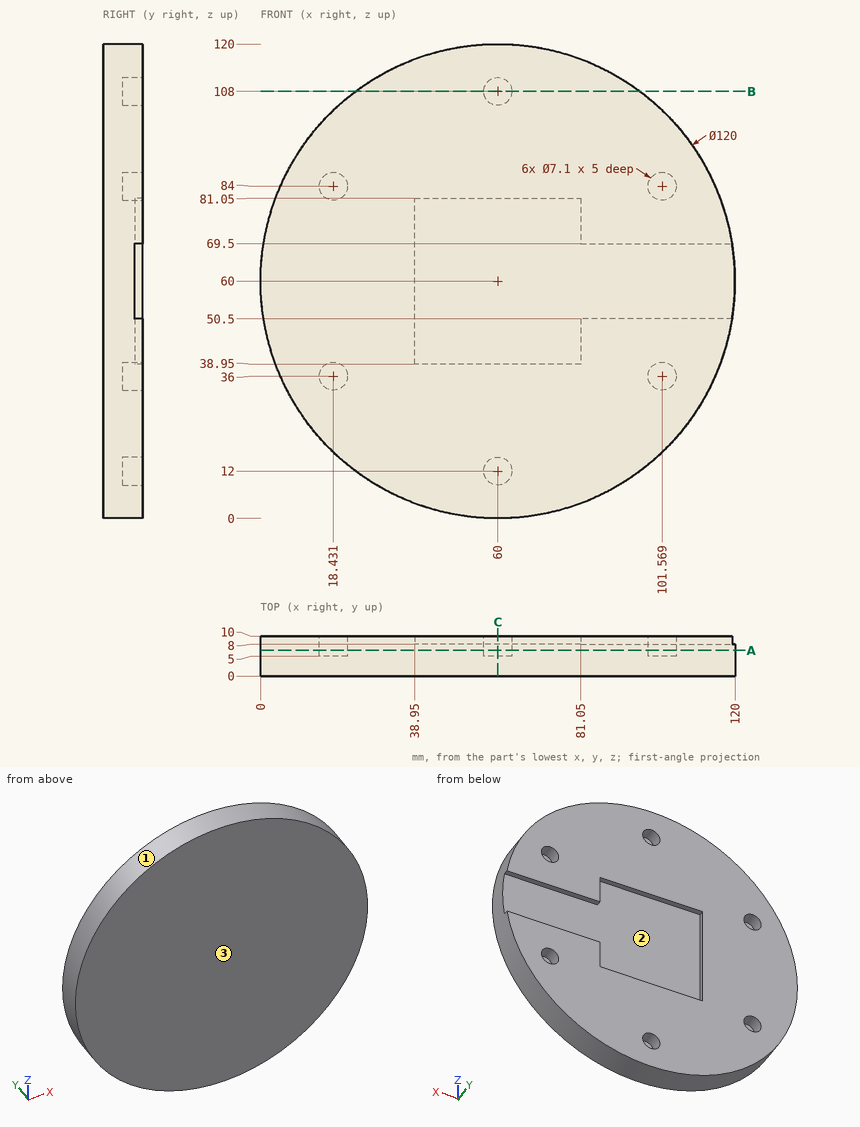
Design review of the part shown in the three views and the two pictorial views. Dimensions are in mm from the part's minimum x, y and z. Give positions to 0.01 mm unless a question says otherwise; leave off trailing zeros. Write each loop counter-clockwise with the first axis right and the second up, starting at its lowest first coordinate (ties: lowest second). Pieces come first, ordered by that corner, then holes. Notation, with made-up numbers: M -35.5,57.5 L 4.5,57.5 A27 ccw 4.5,79.5 Z; hole C 83,40 d10. An arc over 180 degrees is marked long. Answer as CSV lines item,"result".
1. Consider section A-A, the plane y = 6.5. Write out the cut boundary in (x, z), then the cut area to 3 significant figures.
Findings:
outline,"C 60,60 d120; hole C 18.43,36 d7.1; hole C 18.43,84 d7.1; hole C 60,12 d7.1; hole C 60,108 d7.1; hole C 101.57,36 d7.1; hole C 101.57,84 d7.1"
area,"11,100 mm2"
2. Wall thickness on line 1 (X direction, y = 6.8, z = 36); line 2 (X direction, y = 8.25, z = 36.5) (1 decimal); line 3 (Z direction, x = 18, y = 9.25): over which ranges is each line inside the solid? List them lowest first.
Findings:
line 1,"x = 5.01 to 14.88, 21.98 to 98.02, 105.12 to 114.99"
line 2,"x = 4.8 to 14.9, 21.9 to 98.1, 105.1 to 115.2"
line 3,"z = 17.15 to 32.48, 39.52 to 80.48, 87.52 to 102.85"
3. Consider section C-C, the plane x = 60. Write out the cut boundary in (y, z), then the cut area to 3 significant figures.
Findings:
outline,"M 0,0 L 10,0 L 10,8.45 L 5,8.45 L 5,15.55 L 10,15.55 L 10,38.95 L 8,38.95 L 8,81.05 L 10,81.05 L 10,104.45 L 5,104.45 L 5,111.55 L 10,111.55 L 10,120 L 0,120 Z"
area,"1,040 mm2"
4. For pin 1 (1 mm diameter, centred on x = 95.5, y = 9.5, fed in from +Z); pin 2 (0.6 mm diameter, centred on x = 103.5, y = 9.5, fed in from -Z); pin 3 (0.6 mm diameter, centred on y = 9.5, z = 64, fed in from +X), all flat-tipped, find the tip position at first contact; note any pin that passes through.
Findings:
pin 1,"stops at z = 108.73"
pin 2,"stops at z = 18.36"
pin 3,"stops at x = 38.95"
5. Consider section B-B, the plane z = 108. Write out the cut boundary in (x, y).
Findings:
outline,"M 24,0 L 96,0 L 96,10 L 63.55,10 L 63.55,5 L 56.45,5 L 56.45,10 L 24,10 Z"
6. Draft analysis for pull direction Z (two halves, no side actions). For the marked faces 1, 2 and 3, state which applies: +Z half, -Z half, draft (parallel to the pull), parting line (faces both ways), or undercut.
Findings:
face 1,"parting line"
face 2,"undercut"
face 3,"draft"
